Can you work these out from the model? Positions are in its coordinate system, mm. A direction names the side the tool comes from. Coordinates: 2 decimals unless noted, no trailing zeros. Order: outer loops, then holes, each group sorted by start corner. A loop starts at its lowest first (then second) coordinate and runs counter-clockwise, first axis right, second up. Notation, with made-up numbers: (2, 19) -> (45, 19) arc R9 ccw to (45, 28) -> close; hole circle Ø7 at (75.25, 51.5). An arc over 180 degrees is marked (long way). Answer in a Markdown table with one row per item.
```python
from build123d import *

# Parameters (mm, degrees)
SKETCH_1_W      = 15
SKETCH_1_H      = 5
EXTRUDE_1_DEPTH = 3
SKETCH_2_R      = 1.5
EXTRUDE_2_DEPTH = 3
FILLET_2_R      = 1


with BuildPart() as part:
    # 草图1 → 凸台-拉伸1 (new body)
    with BuildSketch(Plane.XY):
        with Locations((-9.275700935, 1.740654206)):
            Rectangle(SKETCH_1_W, SKETCH_1_H)
    extrude(amount=EXTRUDE_1_DEPTH)

    # 草图2 → 凸台-拉伸2 (add)
    with BuildSketch(Plane.XY.offset(3)):
        with Locations((-4.775700935, 1.740654206)):
            Circle(SKETCH_2_R)
    extrude(amount=EXTRUDE_2_DEPTH)

    # 圆角2
    fillet_2_edges = [part.edges().sort_by_distance(p)[0] for p in [
        (-1.775700935, 4.240654206, 1.5),
    ]]
    fillet(fillet_2_edges, radius=FILLET_2_R)


solid = part.part
```
(1) I need wall thicknesses on line 1 (Z direction, x = -6.5, y = 4); line 2 (X direction, y = 3.8, z = 1.8); line 3 (Y direction, x = -5.5, z = 5.55). Which ranges of each line are inside material? Lowest first, please. Write a range as [from, to].
Response values:
| item | result |
|---|---|
| line 1 | [0, 3] |
| line 2 | [-16.78, -1.95] |
| line 3 | [0.43, 3.05] |
(2) Will these pins go through, and if not, where does the flat tip stop? pin 1 Ø1 at (y, z) = (3, 5) entering from -X; pin 2 Ø2.5 at (x, y) = (-12, 2) entering from +Z.
Response values:
| item | result |
|---|---|
| pin 1 | x = -6.07 |
| pin 2 | z = 3 |
(3) Suppose I cut it at B-B (y = 0.5). Please give me the cut outline in (x, z), and give its area (3 significant figures).
Response values:
| item | result |
|---|---|
| outline | (-16.78, 0) -> (-1.78, 0) -> (-1.78, 3) -> (-3.93, 3) -> (-3.93, 6) -> (-5.62, 6) -> (-5.62, 3) -> (-16.78, 3) -> close |
| area | 50.1 mm2 |
(4) Suppose I cut it at D-D (y = -0.2). Please give me the cut outline in (x, z).
Response values:
| item | result |
|---|---|
| outline | (-16.78, 0) -> (-1.78, 0) -> (-1.78, 3) -> (-16.78, 3) -> close |
(5) Suppose I cut it at A-A (x = -4.5). Please give me the cut outline in (y, z).
Response values:
| item | result |
|---|---|
| outline | (-0.76, 0) -> (4.24, 0) -> (4.24, 3) -> (3.22, 3) -> (3.22, 6) -> (0.27, 6) -> (0.27, 3) -> (-0.76, 3) -> close |
(6) On a 3-axis mill with a long thin cutter (end or side, diameter ignored), from which of +Z, -Z, +X, -X, +Y, -Y can I reach the whole of each face in a straight line? I mean faces 1 (the flat face through (-10, 4.241, 1)), 2 (the cylindrical face through (-3.39, 1.17, 4.48)). Say none if no direction works.
Response values:
| item | result |
|---|---|
| face 1 | +Z, -Z, +X, -X, +Y |
| face 2 | +Z |
(7) Suppose I cut it at C-C (z = 4.85). Please give me the cut outline in (x, y).
Response values:
| item | result |
|---|---|
| outline | circle Ø3 at (-4.78, 1.74) |
